```python
from build123d import *

# Parameters (mm, degrees)
SKETCH_1_R          = 1.25
EXTRUDE_1_DEPTH     = 40
SKETCH_2_R          = 1.25
EXTRUDE_2_DEPTH     = 30
SKETCH_2_3_R        = 1.25
CUT_EXTRUDE_1_DEPTH = 10
EXTRUDE_START       = -10
EXTRUDE_3_DEPTH     = 10
CUT_EXTRUDE_START   = -15
SKETCH_4_R          = 1.25
CUT_EXTRUDE_2_DEPTH = 15
SKETCH_5_R          = 1.25
CUT_EXTRUDE_3_DEPTH = 15
EXTRUDE_4_DEPTH     = 40


with BuildPart() as part:
    # 草图1 → 凸台-拉伸1 (new body)
    with BuildSketch(Plane(origin=(0, 0, 0), x_dir=(1, 0, 0), z_dir=(0, 1, 0))):
        Polygon((-3.5, 3.5), (-3.5, -10.5), (1.449747468, -10.5), (7.449747468, -10.5), (13.495730206, -4.454017262), (13.504269794, -4.454017262), (19.550252532, -10.5), (24.5, -10.5), (30.5, -10.5), (30.5, 3.5), (24.5, 3.5), align=None)
        with Locations(Location((0, 0, 0), (0, 0, 270))):
            Circle(SKETCH_1_R, mode=Mode.SUBTRACT)
        with Locations(Location((7, 0, 0), (0, 0, 270))):
            Circle(SKETCH_1_R, mode=Mode.SUBTRACT)
        with Locations(Location((14, 0, 0), (0, 0, 270))):
            Circle(SKETCH_1_R, mode=Mode.SUBTRACT)
        with Locations(Location((21, 0, 0), (0, 0, 270))):
            Circle(SKETCH_1_R, mode=Mode.SUBTRACT)
        with Locations(Location((21, -7, 0), (0, 0, 270))):
            Circle(SKETCH_1_R, mode=Mode.SUBTRACT)
        with Locations(Location((0, -7, 0), (0, 0, 270))):
            Circle(SKETCH_1_R, mode=Mode.SUBTRACT)
    extrude(amount=EXTRUDE_1_DEPTH)

    # 草图2 → 凸台-拉伸2 (add)
    with BuildSketch(Plane.XZ):
        with Locations(Location((0, 7, 0), (0, 0, 270))):
            Circle(SKETCH_2_R)
        with Locations(Location((0, 0, 0), (0, 0, 270))):
            Circle(SKETCH_2_R)
        with Locations((6, 0)):
            Circle(SKETCH_2_R)
        with Locations(Location((7, 0, 0), (0, 0, 270))):
            Circle(SKETCH_2_R)
        with Locations((13, 0)):
            Circle(SKETCH_2_R)
        with Locations(Location((14, 0, 0), (0, 0, 270))):
            Circle(SKETCH_2_R)
        with Locations((20, 0)):
            Circle(SKETCH_2_R)
        with Locations(Location((21, 0, 0), (0, 0, 270))):
            Circle(SKETCH_2_R)
        with Locations(Location((21, 7, 0), (0, 0, 270))):
            Circle(SKETCH_2_R)
    extrude(amount=-EXTRUDE_2_DEPTH)

    # 草图2<3> → 切除-拉伸1 (cut)
    with BuildSketch(Plane.XZ):
        with Locations(Location((27, 7, 0), (0, 0, 270))):
            Circle(SKETCH_2_3_R)
        with Locations(Location((27, 0, 0), (0, 0, 270))):
            Circle(SKETCH_2_3_R)
        with Locations(Location((20, 0, 0), (0, 0, 270))):
            Circle(SKETCH_2_3_R)
        with Locations(Location((13, 0, 0), (0, 0, 270))):
            Circle(SKETCH_2_3_R)
        with Locations(Location((6, 0, 0), (0, 0, 270))):
            Circle(SKETCH_2_3_R)
        with Locations(Location((6, 7, 0), (0, 0, 270))):
            Circle(SKETCH_2_3_R)
    extrude(amount=-CUT_EXTRUDE_1_DEPTH, mode=Mode.SUBTRACT)

    # 草图3 → 凸台-拉伸3 (add)
    with BuildSketch(Plane(origin=(0, 40, 0), x_dir=(1, 0, 0), z_dir=(0, 1, 0)).offset(EXTRUDE_START)):
        with BuildLine():
            ThreePointArc((1.124456691, -6.454017262), (0, -5.75), (-1.124456691, -6.454017262))
            Line((-1.124456691, -6.454017262), (1.124456691, -6.454017262))
        make_face()
        with BuildLine():
            Line((1.124456691, -6.454017262), (-1.124456691, -6.454017262))
            ThreePointArc((-1.124456691, -6.454017262), (-0.280115276, -8.218209929), (1.25, -7))
            ThreePointArc((1.25, -7), (1.218209929, -6.719884724), (1.124456691, -6.454017262))
        make_face()
        with BuildLine():
            ThreePointArc((22.25, -7), (22.218209929, -6.719884724), (22.124456691, -6.454017262))
            Line((22.124456691, -6.454017262), (19.875543309, -6.454017262))
            ThreePointArc((19.875543309, -6.454017262), (20.719884724, -8.218209929), (22.25, -7))
        make_face()
        with BuildLine():
            Line((19.875543309, -6.454017262), (22.124456691, -6.454017262))
            ThreePointArc((22.124456691, -6.454017262), (21, -5.75), (19.875543309, -6.454017262))
        make_face()
    extrude(amount=EXTRUDE_3_DEPTH)

    # 草图4 → 切除-拉伸2 (cut)
    with BuildSketch(Plane(origin=(0, 40, 0), x_dir=(1, 0, 0), z_dir=(0, 1, 0)).offset(CUT_EXTRUDE_START)):
        with Locations(Location((21, 0, 0), (0, 0, 270))):
            Circle(SKETCH_4_R)
        with Locations(Location((14, 0, 0), (0, 0, 270))):
            Circle(SKETCH_4_R)
        with Locations(Location((7, 0, 0), (0, 0, 270))):
            Circle(SKETCH_4_R)
        with Locations(Location((0, 0, 0), (0, 0, 270))):
            Circle(SKETCH_4_R)
    extrude(amount=CUT_EXTRUDE_2_DEPTH, mode=Mode.SUBTRACT)

    # 草图5 → 切除-拉伸3 (cut)
    with BuildSketch(Plane.XZ):
        with Locations(Location((6, 7, 0), (0, 0, 270))):
            Circle(SKETCH_5_R)
        with Locations(Location((27, 7, 0), (0, 0, 270))):
            Circle(SKETCH_5_R)
        with Locations(Location((27, 0, 0), (0, 0, 270))):
            Circle(SKETCH_5_R)
        with Locations(Location((20, 0, 0), (0, 0, 270))):
            Circle(SKETCH_5_R)
        with Locations(Location((13, 0, 0), (0, 0, 270))):
            Circle(SKETCH_5_R)
        with Locations(Location((6, 0, 0), (0, 0, 270))):
            Circle(SKETCH_5_R)
    extrude(amount=-CUT_EXTRUDE_3_DEPTH, mode=Mode.SUBTRACT)

    # 草图6 → 凸台-拉伸4 (add)
    with BuildSketch(Plane(origin=(0, 40, 0), x_dir=(1, 0, 0), z_dir=(0, 1, 0))):
        with BuildLine():
            Line((13.504269794, -4.454017262), (13.495730206, -4.454017262))
            Line((13.495730206, -4.454017262), (9.964466094, -7.985281374))
            ThreePointArc((9.964466094, -7.985281374), (13.5, -6.52081528), (17.035533906, -7.985281374))
            Line((17.035533906, -7.985281374), (13.504269794, -4.454017262))
        make_face()
    extrude(amount=-EXTRUDE_4_DEPTH)


solid = part.part
```
Geometry: final body of the model. Coordinates: model frame, mm. A direction names the side the tool comes from. Give positions to 0.01 mm unless a question says otherwise; leave off trailing zeros. Write each loop counter-clockwise with the first axis right and the second up, starting at its lowest first coordinate (ties: lowest second). Pieces come first, ordered by that corner, then holes.
1. Pin query (flat end, axial travel): P1, Ø2, axis at x = 0, z = 0, coming from the +Y side; P2, Ø1, axis at x = 13.5, z = 0.5, coming from the -Y side; P3, Ø1, axis at x = 18.5, y = 17, coming from the +Z side; P4, Ø4, axis at x = 20, z = 0, coming from the +Y side. Return the tip coordinate at first contact, or that it passes through.
2. Draft query along X for faces 1 (the flat face through (13, 40, 3)), 2 (the flat face through (-3.5, 20, 3)), 3 (the cylindrical face through (18.78, 7.4, 0.27)). Return one class per face: released by +X, released by -X, zero draft, split by the parting line, or undercut.
3. Reachability of faces 4 (the flat face through (18.28, 19.72, 9.23)), 5 (the flat face through (30.5, 20, 4)), 6 (the flat face through (13, 0, 3)), 7 (the flat face through (27, 15, 0)), 8 (the cylindrical face through (5.78, 32.39, -0.27)) from +Z, -Z, +X, -X, +Y, -Y: full face, straight path, thin tool, end or side. Return the list, or none.
4. Section query A-A, the plane y = 29.5. Return loops of the section in (x, z).
5. Line query: probe 1 along X at (y, z) = (8.75, 0); probe 2 along X at (y, z) = (37, 0); probe 3 along X at (y, z) = (8.25, 7). Output: solid intervals per line, ascending.
6. Section query C-C, the plane z = 7. Return loops of the section in (x, y).
7. Section query D-D, the plane y = 18. Return loops of the section in (x, z).
8. Section query B-B, the plane x = 27. Return loops of the section in (y, z).
Computed:
1. P1: stops at y = 25
1. P2: stops at y = 15
1. P3: stops at z = 9.95
1. P4: stops at y = 40
2. face 1: zero draft
2. face 2: released by -X
2. face 3: undercut
3. face 4: +Z, +Y, -Y
3. face 5: +Z, -Z, +X, +Y, -Y
3. face 6: +Z, -Z, +X, -X, -Y
3. face 7: -Y
3. face 8: +Y
4. outline: (-3.5, -3.5) - (30.5, -3.5) - (30.5, 10.5) - (19.55, 10.5) - (17.04, 7.99) arc R5 cw to (9.96, 7.99) - (7.45, 10.5) - (-3.5, 10.5) - close; hole circle Ø2.5 at (0, 0); hole circle Ø2.5 at (7, 0); hole circle Ø2.5 at (14, 0); hole circle Ø2.5 at (21, 0)
5. probe 1: x = -3.5 to 4.75, 7.25 to 11.75, 14.25 to 18.75, 21.25 to 25.75, 28.25 to 30.5
5. probe 2: x = -3.5 to -1.25, 1.25 to 5.75, 8.25 to 12.75, 15.25 to 19.75, 22.25 to 30.5
5. probe 3: x = -3.5 to 4.75, 7.25 to 11.36, 15.64 to 25.75, 28.25 to 30.5
6. outline: (-3.5, 0) - (4.75, 0) - (4.75, 15) - (7.25, 15) - (7.25, 0) - (11.36, 0) - (11.36, 40) - (-3.5, 40) - close; (15.64, 0) - (25.75, 0) - (25.75, 15) - (28.25, 15) - (28.25, 0) - (30.5, 0) - (30.5, 40) - (15.64, 40) - close
7. outline: (-3.5, -3.5) - (30.5, -3.5) - (30.5, 10.5) - (19.55, 10.5) - (17.04, 7.99) arc R5 cw to (9.96, 7.99) - (7.45, 10.5) - (-3.5, 10.5) - close
8. outline: (0, -3.5) - (40, -3.5) - (40, 10.5) - (0, 10.5) - (0, 8.25) - (15, 8.25) - (15, 5.75) - (0, 5.75) - (0, 1.25) - (15, 1.25) - (15, -1.25) - (0, -1.25) - close
